from build123d import *

# Parameters (mm, degrees)
SKETCH_1_R          = 8
EXTRUDE_1_DEPTH     = 6
SKETCH_2_R          = 7
EXTRUDE_2_DEPTH     = 6
SKETCH_4_R          = 3.5
CUT_EXTRUDE_1_DEPTH = 96
CHAMFER_1_SIZE      = 0.5


with BuildPart() as part:
    # Эскиз1 → Вытянуть1 (new body)
    with BuildSketch(Plane.XY):
        Circle(SKETCH_1_R)
    extrude(amount=EXTRUDE_1_DEPTH)

    # Эскиз2 → Вытянуть2 (add)
    with BuildSketch(Plane.XY.offset(6)):
        Circle(SKETCH_2_R)
    extrude(amount=EXTRUDE_2_DEPTH)

    # Эскиз3 → Вырез-Повернуть1 (revolve, cut)
    with BuildSketch(Plane(origin=(0, 0, 0), x_dir=(0, 0, -1), z_dir=(1, 0, 0)), mode=Mode.PRIVATE) as cut_revolve_1_sk:
        with BuildLine():
            Line((-10, 5), (-12, 5))
            Line((-12, 5), (-12, 7))
            Line((-12, 7), (-6.535898385, 7))
            ThreePointArc((-6.535898385, 7), (-8, 5.535898385), (-10, 5))
        make_face()
    revolve(cut_revolve_1_sk.sketch.rotate(Axis((0, 0, 12), (0, 0, -1)), 90), axis=Axis((0, 0, 12), (0, 0, -1)), mode=Mode.SUBTRACT)  # turned: the seam where the file's is

    # Эскиз4 → Вырез-Вытянуть1 (cut)
    with BuildSketch(Plane(origin=(0, 0, 0), x_dir=(-1, 0, 0), z_dir=(0, 0, -1))):
        Circle(SKETCH_4_R)
    extrude(amount=-CUT_EXTRUDE_1_DEPTH, mode=Mode.SUBTRACT)

    # Фаска1
    chamfer_1_edges = [part.edges().sort_by_distance(p)[0] for p in [
        (3.5, 0, 12),
        (3.5, 0, 0),
    ]]
    chamfer(chamfer_1_edges, length=CHAMFER_1_SIZE)


solid = part.part
The model under review builds one solid part; all positions refer to its coordinate system, in mm. A direction names the side the tool comes from. Coordinates: 2 decimals unless noted, no trailing zeros. Write each loop counter-clockwise with the first axis right and the second up, starting at its lowest first coordinate (ties: lowest second). Pieces come first, ordered by that corner, then holes. Notation, with made-up numbers: (8.5, 36) - (57.5, 36) arc R20 ccw to (57.5, 66) - close; hole circle Ø5 at (77, 61.5). An arc over 180 degrees is marked (long way). Answer as a JSON object with one key per item and string values. Group by question number.
1. Clearance check with flat-ended pins moving along their axes: pin 1 Ø1 at (y, z) = (-5.5, 5) entering from +X (3 decimals); pin 2 Ø3 at (y, z) = (-5, 5) entering from -X; pin 3 Ø4 at (x, z) = (3, 2) entering from +Y. State where each tip first meets the part, or that it passes through.
2. Machinability: for faces 1 (the face through (-5, 0, 11)), 2 (the face through (-3.233, -1.341, 5.923)), which of the approach directions +Z, -Z, +X, -X, +Y, -Y give a long, thin tool a straight path to every point of the face, cutting with its end or side? Answer none if there is none.
3. To check wall thickness, follow probe 1 along Y at (x, z) = (0, 4); probe 2 along X at (y, z) = (-1.5, 7); probe 3 along X at (y, z) = (-2.75, 2). State the ranges of each line that lie inside material, in increasing order.
4. Add section D-D (z = 11). Give the boundary of the cut face in (x, y).
5. Add section A-A (y = 0). Give the boundary of the cut face in (x, z), plus the area to 3 significant figures.
6. Add section C-C (z = 2). Give the boundary of the cut face in (x, y).
Findings:
{
 "1": {"pin 1": "x = 6.245", "pin 2": "x = -7.19", "pin 3": "y = 7.94"},
 "2": {"face 1": "+Z", "face 2": "+Z, -Z"},
 "3": {"probe 1": "-8 to -3.5, 3.5 to 8", "probe 2": "-6.17 to -3.16, 3.16 to 6.17", "probe 3": "-7.51 to -2.17, 2.17 to 7.51"},
 "4": {"outline": "circle Ø10 at (0, 0); hole circle Ø7 at (0, 0)"},
 "5": {"outline": "(-8, 0) - (-4, 0) - (-3.5, 0.5) - (-3.5, 11.5) - (-4, 12) - (-5, 12) - (-5, 10) arc R4 cw to (-7, 6.54) - (-7, 6) - (-8, 6) - close; (3.5, 0.5) - (4, 0) - (8, 0) - (8, 6) - (7, 6) - (7, 6.54) arc R4 cw to (5, 10) - (5, 12) - (4, 12) - (3.5, 11.5) - close", "area": "77.7 mm²"},
 "6": {"outline": "circle Ø16 at (0, 0); hole circle Ø7 at (0, 0)"}
}
